from build123d import *

# Parameters (mm, degrees)
SKETCH1_W           = 30
SKETCH1_H           = 40
BOSS_EXTRUDE1_DEPTH = 5
BOSS_EXTRUDE2_DEPTH = 5
FILLET1_R           = 5
CUT_EXTRUDE1_DEPTH  = 5


with BuildPart() as part:
    # Sketch1 → Boss-Extrude1 (new body)
    with BuildSketch(Plane.XY):
        Rectangle(SKETCH1_W, SKETCH1_H)
    extrude(amount=BOSS_EXTRUDE1_DEPTH)

    # Sketch2 → Boss-Extrude2 (add)
    with BuildSketch(Plane(origin=(0, 20, 0), x_dir=(1, 0, 0), z_dir=(0, 1, 0))):
        Polygon((-15, -5), (64.346756059, -42), (15, -5), align=None)
    extrude(amount=-BOSS_EXTRUDE2_DEPTH)

    # Fillet1
    fillet1_edges = [part.edges().sort_by_distance(p)[0] for p in [
        (15, -20, 2.5),
        (-15, -20, 2.5),
    ]]
    fillet(fillet1_edges, radius=FILLET1_R)

    # Sketch3 → Cut-Extrude1 (cut)
    with BuildSketch(Plane(origin=(0, 0, 0), x_dir=(-1, 0, 0), z_dir=(0, 0, -1))):
        with BuildLine():
            Line((7.5, -13.1), (-7.5, -13.1))
            ThreePointArc((-7.5, -13.1), (-9.6, -11), (-7.5, -8.9))
            Line((-7.5, -8.9), (7.5, -8.9))
            ThreePointArc((7.5, -8.9), (9.6, -11), (7.5, -13.1))
        make_face()
    extrude(amount=-CUT_EXTRUDE1_DEPTH, mode=Mode.SUBTRACT)


solid = part.part
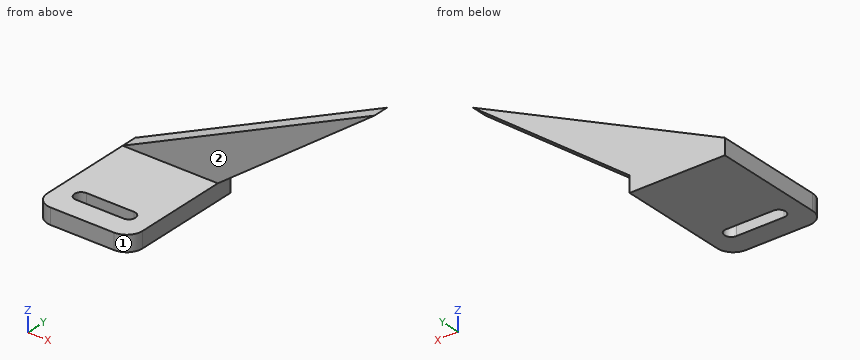
Part model, mm, in its own coordinate system. Face numbers are marked on the shaded views. A direction names the side the tool comes from. Coordinates: 2 decimals unless noted, no trailing zeros. Order: outer loops, then holes, each group sorted by start corner. A loop starts at its lowest first (then second) coordinate and runs counter-clockwise, first axis right, second up. Notation, with made-up numbers: M -16.5,53.25 L 1.5,53.25 A25 cw 1.5,75.25 Z; hole C 26.5,29 d8. An arc over 180 degrees is marked long. Use a Markdown table: item, result.
(1) Probe L1, parallel to Z at x = 5, y = 8.5; L2, parallel to X at y = 7, z = 2.5; L3, parallel to Y at x = 56, z = 38. List the from-to ranges inside material, lowest first.
A:
| item | result |
|---|---|
| L1 | z = 0 to 5 |
| L2 | x = -15 to 15 |
| L3 | y = 15 to 20 |
(2) Cut at C-C on y = 8. Write the cut outline in (x, z).
A:
| item | result |
|---|---|
| outline | M -15,0 L 15,0 L 15,5 L -15,5 Z |
(3) Cut at D-D on x = 3. Write the cut outline in (y, z).
A:
| item | result |
|---|---|
| outline | M -20,0 L -13.1,0 L -13.1,5 L -20,5 Z; M -8.9,0 L 20,0 L 20,13.39 L 15,13.39 L 15,5 L -8.9,5 Z |
(4) Cut at B-B on x = -6. Write the cut outline in (y, z).
A:
| item | result |
|---|---|
| outline | M -20,0 L -13.1,0 L -13.1,5 L -20,5 Z; M -8.9,0 L 20,0 L 20,9.2 L 15,9.2 L 15,5 L -8.9,5 Z |
(5) Tool access for the marked faces 1 and 2: list every direction of +Z, -Z, +X, -X, +Y, -Y with a clear straight run to the whole face (end or side of a thin tool).
A:
| item | result |
|---|---|
| face 1 | +Z, -Z, +X, -Y |
| face 2 | +Z, +X, -X, -Y |
(6) Flat gauge pins, fed straight in: pin 1 (4 mm diameter, centred on x = 28, z = 19, fed in from -Y); pin 2 (12 mm diameter, centred on y = 12, z = 13.5, fed in from -X); pin 3 (2.5 mm diameter, centred on y = -3, z = 3, fed in from +X). Where does each tip first touch, or does it go through?
A:
| item | result |
|---|---|
| pin 1 | stops at y = 15 |
| pin 2 | stops at x = -7.91 |
| pin 3 | stops at x = 15 |
(7) Cut at A-A on y = -11. Write the cut outline in (x, z).
A:
| item | result |
|---|---|
| outline | M -15,0 L -9.6,0 L -9.6,5 L -15,5 Z; M 9.6,0 L 15,0 L 15,5 L 9.6,5 Z |
